```python
from build123d import *

# Parameters (mm, degrees)
SKETCH1_W                = 6
SKETCH1_H                = 1.2
SKETCH1_W_2              = 1.2
SKETCH1_H_2              = 5.4
REVOLVE1_ANGLE           = 180
REVOLVE2_START           = 5.4
REVOLVE2_DEPTH           = 1.6
SKETCH4_W                = 6.4
SKETCH4_H                = 2
CUT_EXTRUDE1_DEPTH       = 10
SKETCH5_R                = 3
CUT_EXTRUDE2_DEPTH       = 10
SKETCH6_W                = 2.4
SKETCH6_H                = 1.5
BOSS_EXTRUDE1_DEPTH      = 1.2
SKETCH7_W                = 1.2
SKETCH7_H                = 2.9
BOSS_EXTRUDE2_DEPTH      = 1.7
CHAMFER1_SIZE            = 0.5
CHAMFER1_OF_MIRROR1_SIZE = 0.5


# Read off the part's stored shape, not the designer's step: Revolve2
with BuildPart() as part:
    # Sketch1 → Revolve1 (revolve)
    with BuildSketch(Plane.XY):
        with Locations((3, -0.6)):
            Rectangle(SKETCH1_W, SKETCH1_H)
        with Locations((6.6, -0.6)):
            Rectangle(SKETCH1_W_2, SKETCH1_H)
        with Locations((6.6, 2.7)):
            Rectangle(SKETCH1_W_2, SKETCH1_H_2)
    revolve(axis=Axis((0, -1.2, 0), (0, 1, 0)), revolution_arc=REVOLVE1_ANGLE)

    # Revolve2 outline → Revolve2 (add)
    with BuildSketch(Plane(origin=(0, 0, 0), x_dir=(1, 0, 0), z_dir=(0, 1, 0)).offset(REVOLVE2_START)):
        with BuildLine():
            ThreePointArc((3.65, 6.206246853), (0, 7.2), (-3.65, 6.206246853))
            Line((-3.65, 6.206246853), (-3.65, 4.762089877))
            ThreePointArc((-3.65, 4.762089877), (0, 6), (3.65, 4.762089877))
            Line((3.65, 4.762089877), (3.65, 6.206246853))
        make_face()
    extrude(amount=REVOLVE2_DEPTH)

    # Sketch4 → Cut-Extrude1 (cut)
    with BuildSketch(Plane.XY):
        with Locations((0, 1.8)):
            Rectangle(SKETCH4_W, SKETCH4_H)
    extrude(amount=-CUT_EXTRUDE1_DEPTH, mode=Mode.SUBTRACT)

    # Sketch5 → Cut-Extrude2 (cut)
    with BuildSketch(Plane(origin=(0, 0, 0), x_dir=(1, 0, 0), z_dir=(0, 1, 0))):
        Circle(SKETCH5_R)
    extrude(amount=-CUT_EXTRUDE2_DEPTH, mode=Mode.SUBTRACT)

    # Sketch6 → Boss-Extrude1 (add)
    with BuildSketch(Plane(origin=(0, 0, 0), x_dir=(1, 0, 0), z_dir=(0, 1, 0))):
        with Locations((-4.2, -0.75)):
            Rectangle(SKETCH6_W, SKETCH6_H)
    boss_extrude1 = extrude(amount=-BOSS_EXTRUDE1_DEPTH)

    # Sketch7 → Boss-Extrude2 (add)
    with BuildSketch(Plane(origin=(-6, 0, 0), x_dir=(0, 0, -1), z_dir=(1, 0, 0))):
        with Locations((-0.6, 2.1)):
            Rectangle(SKETCH7_W, SKETCH7_H)
    boss_extrude2 = extrude(amount=-BOSS_EXTRUDE2_DEPTH)

    # Chamfer1
    chamfer1_edges = [part.edges().sort_by_distance(p)[0] for p in [
        (-7.7, 2.1, 1.2),
    ]]
    chamfer(chamfer1_edges, length=CHAMFER1_SIZE)

    # Mirror1: Boss-Extrude1, Boss-Extrude2 across plane
    add(boss_extrude1.mirror(Plane(origin=(0, 0, 0), x_dir=(0, 0, 1), z_dir=(1, 0, 0))))
    add(boss_extrude2.mirror(Plane(origin=(0, 0, 0), x_dir=(0, 0, 1), z_dir=(1, 0, 0))))

    # Chamfer1 of Mirror1
    chamfer1_of_mirror1_edges = [part.edges().sort_by_distance(p)[0] for p in [
        (7.7, 2.1, 1.2),
    ]]
    chamfer(chamfer1_of_mirror1_edges, length=CHAMFER1_OF_MIRROR1_SIZE)


solid = part.part
```
Check sheet for the modelled part. Datum: model origin and axes. Units: mm. A direction names the side the tool comes from. Round coordinates to 2 decimals unless told otherwise and drop trailing zeros. Order: outer loops, then holes, each group sorted by start corner. A loop starts at its lowest first (then second) coordinate and runs counter-clockwise, first axis right, second up. Notation, with made-up numbers: (5.5, 55.5) -> (48.5, 55.5) arc R20 cw to (48.5, 70.5) -> close; hole circle Ø1 at (69, 86.25). An arc over 180 degrees is marked (long way). One line per item, written item: value. Start each with the question number.
Q1. Cross-section at C-C (z = -0.25). Record the boundary of the cut face in (x, y), and give its area (3 significant figures).
Q2. Cross-section at B-B (x = 0). Record the boundary of the cut face in (y, z).
Q3. Cross-section at A-A (y = 2.5). Record the boundary of the cut face in (x, z).
Q4. Gauge pin test, flat ends, axial feed: pin 1 Ø0.6 at (y, z) = (-0.5, 0.5) entering from +X; pin 2 Ø3 at (x, y) = (5, 0) entering from -Z; pin 3 Ø0.7 at (y, z) = (6.5, -5.5) entering from +X. Record the tip position at first contact, or that the pin passes through.
Q5. Cross-section at D-D (y = -0.5). Record the boundary of the cut face in (x, z).
Q6. Set-up check for faces 1 (the face through (-6, 2, 1)), 2 (the face through (3.65, 6, -5)), 3 (the face through (-7, 0.65, 1)): record each of +Z, -Z, +X, -X, +Y, -Y from which the full face is reachable in a straight line by a thin tool's end or side.
Q7. Thickness scan on line 1 (Y direction, x = 5.25, z = 0.75); line 2 (X direction, y = 0.5, z = -2.5); line 3 (X direction, y = 5, z = -4). Record the ranges inside material, lowest first.
Q8. Mould release check, pull along X, two halves, no side actions. Record for faces 4 (the face through (-5.4, -1, 1)), 5 (the face through (3.2, 2, -6)), 6 (the face through (3, -1, 1)), 7 (the face through (-0.1, 7, -6.3)): pulls with the +X half, pulls with the -X half, needs draft (parallel to the pull), parting line crosses it, or undercut.
Completed:
1. outline: (-7.2, -1.2) -> (-2.99, -1.2) -> (-2.99, 0) -> (-5.99, 0) -> (-5.99, 5.4) -> (-7.2, 5.4) -> close; (2.99, -1.2) -> (7.2, -1.2) -> (7.2, 5.4) -> (5.99, 5.4) -> (5.99, 0) -> (2.99, 0) -> close
1. area: 23.1 mm²
2. outline: (-1.2, -7.2) -> (0.8, -7.2) -> (0.8, -6) -> (0, -6) -> (0, -3) -> (-1.2, -3) -> close; (2.8, -7.2) -> (7, -7.2) -> (7, -6) -> (2.8, -6) -> close
3. outline: (-7.7, 0) -> (-7.2, 0) arc R7.2 ccw to (-3.2, -6.45) -> (-3.2, -5.08) arc R6 cw to (-6, 0) -> (-6, 1.2) -> (-7.2, 1.2) -> (-7.7, 0.7) -> close; (3.2, -6.45) arc R7.2 ccw to (7.2, 0) -> (7.7, 0) -> (7.7, 0.7) -> (7.2, 1.2) -> (6, 1.2) -> (6, 0) arc R6 cw to (3.2, -5.08) -> close
4. pin 1: stops at x = 5.4
4. pin 2: stops at z = -6.29
4. pin 3: stops at x = 3.65
5. outline: (-7.2, 0) arc R7.2 ccw to (7.2, 0) -> (5.4, 0) -> (5.4, 1.5) -> (3, 1.5) -> (3, 0) arc R3 cw to (-3, 0) -> (-3, 1.5) -> (-5.4, 1.5) -> (-5.4, 0) -> close
6. face 1: +Z, +Y, -Y
6. face 2: +Z, -Z, +X, +Y
6. face 3: +Z, +X, -X, -Y
7. line 1: y = -1.2 to 0
7. line 2: x = -6.75 to -5.45, 5.45 to 6.75
7. line 3: x = -5.99 to -4.47, 4.47 to 5.99
8. face 4: pulls with the -X half
8. face 5: undercut
8. face 6: undercut
8. face 7: needs draft
